```python
from build123d import *

# Parameters (mm, degrees)
BASE_FACE_R         = 4
BASE_FACE_R_2       = 1.5
BASE_DEPTH          = 3.3
SKETCH3_W           = 26.5
SKETCH3_H           = 33
SKETCH3_R           = 4.9
SKETCH3_R_2         = 1.65
BOSS_EXTRUDE2_DEPTH = 3.3
FILLET1_R           = 2


with BuildPart() as part:
    # Base Face → Base (new body)
    with BuildSketch(Plane(origin=(0, 0, 0), x_dir=(1, 0, 0), z_dir=(0, 1, 0))):
        with BuildLine():
            Line((-13.25, 0), (-13.25, -20.75))
            Line((-13.25, -20.75), (13.25, -20.75))
            Line((13.25, -20.75), (13.25, 0))
            ThreePointArc((13.25, 0), (0, 13.25), (-13.25, 0))
        make_face()
        Circle(BASE_FACE_R, mode=Mode.SUBTRACT)
        with Locations((-8.5, 0)):
            Circle(BASE_FACE_R_2, mode=Mode.SUBTRACT)
        with Locations((8.5, 0)):
            Circle(BASE_FACE_R_2, mode=Mode.SUBTRACT)
    extrude(amount=BASE_DEPTH)

    # Sketch3 → Boss-Extrude2 (add)
    with BuildSketch(Plane.XY.offset(20.75)):
        with Locations((0, 16.5)):
            Rectangle(SKETCH3_W, SKETCH3_H)
        with Locations((0, 17.8)):
            Circle(SKETCH3_R, mode=Mode.SUBTRACT)
        with Locations((8, 10.85)):
            Circle(SKETCH3_R_2, mode=Mode.SUBTRACT)
        with Locations((8, 24.85)):
            Circle(SKETCH3_R_2, mode=Mode.SUBTRACT)
        with Locations((-8, 10.85)):
            Circle(SKETCH3_R_2, mode=Mode.SUBTRACT)
        with Locations((-8, 24.85)):
            Circle(SKETCH3_R_2, mode=Mode.SUBTRACT)
    extrude(amount=-BOSS_EXTRUDE2_DEPTH)

    # Fillet1
    fillet1_edges = [part.edges().sort_by_distance(p)[0] for p in [
        (0, 0, 20.75),
    ]]
    fillet(fillet1_edges, radius=FILLET1_R)


solid = part.part
```
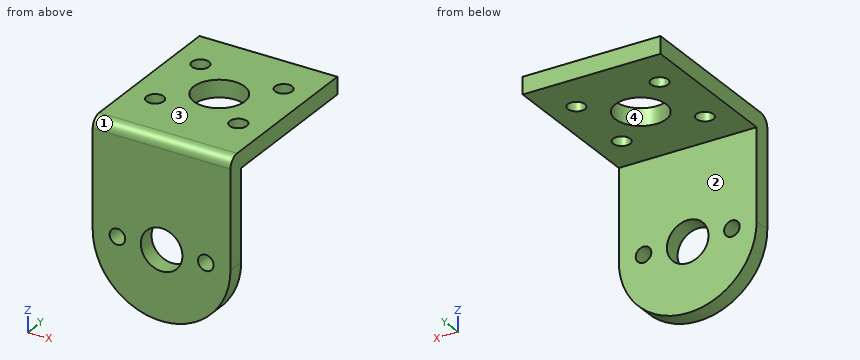
Read the model definition and answer for the solid it produces. Units are mm, in the model's axes. Face numbers are marked on the shaded views. A direction names the side the tool comes from. Coordinates: 2 decimals unless noted, no trailing zeros. Loops run counter-clockwise (first coordinate to the right, second up) from the corner with the lowest first, then second, coordinate; pieces in that order, holes last. Notation, with made-up numbers: (-31.5, -9.5) -> (27.5, -9.5) arc R20 ccw to (27.5, -4.5) -> close; hole circle Ø2 at (32.5, 55.25). An arc over 180 degrees is marked (long way). Return JSON: item names as keys, results as strings.
Item 1: Find section C-C (y = 22). Determine the outline of the cut face in (x, z), plus the area to 3 significant figures.
Answers:
{"outline": "(-13.25, 17.45) -> (-2.52, 17.45) -> (-2.52, 20.75) -> (-13.25, 20.75) -> close; (2.52, 17.45) -> (13.25, 17.45) -> (13.25, 20.75) -> (2.52, 20.75) -> close", "area": "70.8 mm2"}
Item 2: Flat-ended cylindrical pins translate along their axes: P1, Ø5, axis at y = 22.5, z = 14, coming from the -X side; P2, Ø9, axis at x = 0, z = 0, coming from the +Y side; P3, Ø8, axis at x = -2, y = 16.5, coming from the -Z side. Find the tip coordinate at first contact, or state that the pin passes through.
Answers:
{"P1": "passes through", "P2": "stops at y = 3.3", "P3": "stops at z = 17.45"}
Item 3: For a pull along X with two mould halves and no side action, classify the marked faces 3 and 4 as +X half, -X half, draft (parallel to the pull), parting line (faces both ways), or undercut.
Answers:
{"face 3": "draft", "face 4": "undercut"}
Item 4: For the marked faces 1 and 2, determine the directions among +Z, -Z, +X, -X, +Y, -Y from which every point of the face is accessible in a straight line to the end or side of a thin tool.
Answers:
{"face 1": "+Z, +X, -X, -Y", "face 2": "-Z, +X, -X, +Y"}
Item 5: Find section B-B (x = 1). Determine the outline of the cut face in (y, z).
Answers:
{"outline": "(0, -13.21) -> (3.3, -13.21) -> (3.3, -3.87) -> (0, -3.87) -> close; (0, 3.87) -> (3.3, 3.87) -> (3.3, 17.45) -> (13, 17.45) -> (13, 20.75) -> (2, 20.75) arc R2 ccw to (0, 18.75) -> close; (22.6, 17.45) -> (33, 17.45) -> (33, 20.75) -> (22.6, 20.75) -> close"}
Item 6: Find section A-A (y = 10.85). Determine the outline of the cut face in (x, z), plus the area to 3 significant figures.
Answers:
{"outline": "(-13.25, 17.45) -> (-9.65, 17.45) -> (-9.65, 20.75) -> (-13.25, 20.75) -> close; (-6.35, 17.45) -> (6.35, 17.45) -> (6.35, 20.75) -> (-6.35, 20.75) -> close; (9.65, 17.45) -> (13.25, 17.45) -> (13.25, 20.75) -> (9.65, 20.75) -> close", "area": "65.7 mm2"}
Item 7: Find section D-D (x = -8). Determine the outline of the cut face in (y, z).
Answers:
{"outline": "(0, -10.56) -> (3.3, -10.56) -> (3.3, -1.41) -> (0, -1.41) -> close; (0, 1.41) -> (3.3, 1.41) -> (3.3, 17.45) -> (9.2, 17.45) -> (9.2, 20.75) -> (2, 20.75) arc R2 ccw to (0, 18.75) -> close; (12.5, 17.45) -> (23.2, 17.45) -> (23.2, 20.75) -> (12.5, 20.75) -> close; (26.5, 17.45) -> (33, 17.45) -> (33, 20.75) -> (26.5, 20.75) -> close"}
Item 8: Find the intervals of material crossed by probe 1 along X at (y, z) = (1, 0); probe 2 along X at (y, z) = (24, 19); probe 3 along Y at (x, z) = (-8, 19.35), in increasing order.
Answers:
{"probe 1": "x = -13.25 to -10, -7 to -4, 4 to 7, 10 to 13.25", "probe 2": "x = -13.25 to -9.41, -6.59 to 6.59, 9.41 to 13.25", "probe 3": "y = 0.09 to 9.2, 12.5 to 23.2, 26.5 to 33"}
